```python
from build123d import *

# Parameters (mm, degrees)
SKETCH1_R               = 36.83
BOSS_EXTRUDE1_DEPTH     = 22.86
FILLET1_R               = 2.54
SKETCH2_R               = 26.67
SKETCH3_R               = 14.7955
SKETCH4_R               = 14.7955
CUT_EXTRUDE1_DEPTH      = 76.2
SKETCH18_R              = 3.175
CUT_EXTRUDE2_DEPTH      = 6.35
CUT_EXTRUDE3_DEPTH      = 6.35
CUT_EXTRUDE4_START      = 2.54
CUT_EXTRUDE4_DEPTH      = 2.54
CIRPATTERN1_COUNT       = 2
CUT_EXTRUDE5_DEPTH      = 57.881257188
CUT_EXTRUDE5_DEPTH_BACK = 57.881257188
SKETCH22_R              = 3.81


with BuildPart() as part:
    # Sketch1 → Boss-Extrude1 (new body)
    with BuildSketch(Plane(origin=(0, 0, 0), x_dir=(1, 0, 0), z_dir=(0, 1, 0))):
        with Locations(Location((0, 0, 0), (0, 0, 270))):
            Circle(SKETCH1_R)
    extrude(amount=BOSS_EXTRUDE1_DEPTH)

    # Fillet1
    fillet1_edges = [part.edges().sort_by_distance(p)[0] for p in [
        (0, 0, -36.83),
    ]]
    fillet(fillet1_edges, radius=FILLET1_R)

    # Sketch2 → Cut-Loft1 section 0
    with BuildSketch(Plane(origin=(0, 0, 0), x_dir=(1, 0, 0), z_dir=(0, 1, 0))):
        Circle(SKETCH2_R)
    # Sketch3 → Cut-Loft1 section 1
    with BuildSketch(Plane(origin=(0, 11.938, 0), x_dir=(1, 0, 0), z_dir=(0, 1, 0))):
        Circle(SKETCH3_R)
    loft(mode=Mode.SUBTRACT)

    # Sketch4 → Cut-Extrude1 (cut)
    with BuildSketch(Plane.XZ.offset(-11.938)):
        with Locations(Location((0, 0, 0), (0, 0, 270))):
            Circle(SKETCH4_R)
    extrude(amount=-CUT_EXTRUDE1_DEPTH, mode=Mode.SUBTRACT)

    # Sketch17 → Cut-Revolve1 (revolve, cut)
    with BuildSketch(Plane(origin=(0, 0, 0), x_dir=(0, 0, -1), z_dir=(1, 0, 0))):
        with BuildLine():
            Line((36.83, 22.86), (14.7955, 22.86))
            Line((14.7955, 22.86), (14.7955, 17.78))
            ThreePointArc((14.7955, 17.78), (26.280325712, 18.29189035), (36.83, 22.86))
        make_face()
    revolve(axis=Axis((0, 0, 0), (0, 1, 0)), mode=Mode.SUBTRACT)

    # Sketch18 → Cut-Extrude2 (cut)
    with BuildSketch(Plane.XZ):
        with Locations(Location((0, 30.431156816, 0), (0, 0, 270))):
            Circle(SKETCH18_R)
        with Locations(Location((0, -30.431156816, 0), (0, 0, 270))):
            Circle(SKETCH18_R)
    extrude(amount=-CUT_EXTRUDE2_DEPTH, mode=Mode.SUBTRACT)

    # Sketch19 → Cut-Extrude3 (cut)
    with BuildSketch(Plane.XZ):
        with BuildLine():
            Line((4.259709497, -31.701156816), (2.909935566, -31.701156816))
            ThreePointArc((2.909935566, -31.701156816), (3.175, -30.431156816), (2.909935566, -29.161156816))
            Line((2.909935566, -29.161156816), (4.259709497, -29.161156816))
            ThreePointArc((4.259709497, -29.161156816), (4.445, -30.431156816), (4.259709497, -31.701156816))
        make_face()
    cut_extrude3 = extrude(amount=-CUT_EXTRUDE3_DEPTH, mode=Mode.SUBTRACT)

    # Sketch20 → Cut-Extrude4 (cut)
    with BuildSketch(Plane.XZ.offset(-6.35).offset(CUT_EXTRUDE4_START)):
        with BuildLine():
            Line((-1.27, -34.690866313), (-1.27, -33.341092382))
            ThreePointArc((-1.27, -33.341092382), (1.15960956, -33.3868176), (2.909935566, -31.701156816))
            Line((2.909935566, -31.701156816), (4.259709497, -31.701156816))
            ThreePointArc((4.259709497, -31.701156816), (2.114043859, -34.341251899), (-1.27, -34.690866313))
        make_face()
    cut_extrude4 = extrude(amount=-CUT_EXTRUDE4_DEPTH, mode=Mode.SUBTRACT)

    # CirPattern1: Cut-Extrude3, Cut-Extrude4 ×2 about axis
    cirpattern1_axis = Axis((0, 0, 0), (0, 1, 0))
    add([cut_extrude3.rotate(cirpattern1_axis, i * 360 / CIRPATTERN1_COUNT) for i in range(1, CIRPATTERN1_COUNT)], mode=Mode.SUBTRACT)
    add([cut_extrude4.rotate(cirpattern1_axis, i * 360 / CIRPATTERN1_COUNT) for i in range(1, CIRPATTERN1_COUNT)], mode=Mode.SUBTRACT)

    # Sketch22 → Cut-Extrude5 (cut, two sides: drawn at the far end of the back side and taken through both)
    with BuildSketch(Plane(origin=(0, 0, 0), x_dir=(0, 0, -1), z_dir=(1, 0, 0)).offset(-CUT_EXTRUDE5_DEPTH_BACK)):
        with Locations((0, 7.62)):
            Circle(SKETCH22_R)
    extrude(amount=CUT_EXTRUDE5_DEPTH + CUT_EXTRUDE5_DEPTH_BACK, mode=Mode.SUBTRACT)


solid = part.part
```
CAD build for the part. Positions are in the model's coordinates, mm. A direction names the side the tool comes from. Coordinates: 2 decimals unless noted, no trailing zeros. Write each loop counter-clockwise with the first axis right and the second up, starting at its lowest first coordinate (ties: lowest second). Pieces come first, ordered by that corner, then holes.
(1) Two-plate mould, pull along Y, no slides. Class faces 1 (the face through (14.66, 11.36, -4.62)), 2 (the face through (-2, 3.81, 34)), 3 (the face through (2, 3.81, -34)): +Y half, -Y half, draft (parallel to the pull), parting line (faces both ways), or undercut.
(2) Drill centre lines: probe 1 along Z at (x, y) = (0, 5); probe 2 along X at (y, z) = (16.3, 0); probe 3 along Z at (x, y) = (-0.5, 13.75). Where is each one in solid material? Low to high.
(3) 3-axis set-ups, long thin cutter, end or side, ignore diameter. For faces 4 (the face through (28.308, 11.398, 0.496)), 5 (the face through (2.537, 3.131, 28.523)), 6 (the face through (-1, 6.35, 31)): which of +Z, -Z, +X, -X, +Y, -Y reach the whole face in a straight line?
(4) Flat gauge pins, fed straight in: pin 1 (4 mm diameter, centred on x = 0, z = -30.43, fed in from +Y); pin 2 (3 mm diameter, centred on x = 8.5, y = 11, fed in from +Z); pin 3 (2.5 mm diameter, centred on x = 2.5, z = -33, fed in from +Y); pin 4 (4.5 mm diameter, centred on y = 7.62, z = 0, fed in from +X). Where does each tip first touch, or does it go through?
(5) Cut at B-B, the plane z = 0. Count the separate pieces of the cut face and the enclosed holes in it, and give its area (3 significant figures).
(6) Cut at A-A, the plane y = 10.5. List the corners of the cut face in (x, z).
Geometry says:
1. face 1: -Y half
1. face 2: undercut
1. face 3: undercut
2. probe 1: z = -36.83 to -34.88, -27.26 to -21.7, 21.7 to 27.26, 34.88 to 36.83
2. probe 2: x = -36.83 to -14.8, 14.8 to 36.83
2. probe 3: z = -36.83 to -14.79, 14.79 to 36.83
3. face 4: +X, -X
3. face 5: -Y
3. face 6: none
4. pin 1: stops at y = 20.39
4. pin 2: stops at z = 36.16
4. pin 3: stops at y = 21.35
4. pin 4: passes through
5. separate pieces: 4
5. enclosed holes: 0
5. area: 417 mm2
6. outline: (-36.75, -2.49) arc R36.83 ccw to (36.75, -2.49) - (16.03, -2.49) arc R16.23 cw to (-16.03, -2.49) - close; (-36.75, 2.49) - (-16.03, 2.49) arc R16.23 cw to (16.03, 2.49) - (36.75, 2.49) arc R36.83 ccw to start
